Design review of the part built by this model. Coordinates are the model's own, in mm. A direction names the side the tool comes from. Give positions to 0.01 mm unless a question says otherwise; leave off trailing zeros. Loops run counter-clockwise (first coordinate to the right, second up) from the corner with the lowest first, then second, coordinate; pieces in that order, holes last.
Autodesk Inventor part; units mm, degrees
ref_plane "YZ Plane" through (0, 0, 0) normal (1, 0, 0) x (0, 1, 0)
ref_plane "XZ Plane" through (0, 0, 0) normal (0, 1, 0) x (-1, 0, 0)
ref_plane "XY Plane" through (0, 0, 0) normal (0, 0, 1) x (1, 0, 0)
sketch "Sketch1" plane through (0, 0, 0) normal (0, 1, 0) x (-1, 0, 0)
  line L0 (0, 0) -> (2500, 0)
  line L1 (2500, 0) -> (2500, -1250)
  line L2 (2500, -1250) -> (0, -1250)
  line L3 (0, -1250) -> (0, 0)
  dimension "d0" = 2500
  dimension "d1" = 1250
extrude "Extrusion1" add sketch "Sketch1" along normal blind 600
sketch "Sketch2" plane through (0, 0, 0) normal (0, -1, 0) x (1, 0, 0)
  line L0 (-50, -50) -> (-2450, -50)
  line L1 (-2450, -50) -> (-2450, -1200)
  line L2 (-2450, -1200) -> (-50, -1200)
  line L3 (-50, -1200) -> (-50, -50)
  line L4 (0, 0) -> (-2500, 0)
  line L5 (0, -1250) -> (0, 0)
  dimension "d4" = 2400
  dimension "d5" = 1150
  dimension "d8" = 50
  dimension "d9" = 50
  dimension "d10" = 2500
  dimension "d11" = 1250
extrude "Extrusion2" cut sketch "Sketch2" against normal blind 500
sketch "Sketch3" plane through (-2500, 0, 0) normal (0, 0, 1) x (1, 0, 0)
  line L0 (2500, 0) -> (0, 0)
  line L1 (2500, 0) -> (2500, 600)
  line L2 (0, 0) -> (0, 600)
  circle A0 centre (2476, 24) radius 4
  circle A1 centre (2460, 24) radius 4
  dimension "d12" = 8
  dimension "d13" = 24
  dimension "d14" = 24
  dimension "d20" = 8
  dimension "d21" = 24
  dimension "d23" = 16
extrude "Extrusion3" cut sketch "Sketch3" against normal blind 10
ref_plane "Work Plane1" through (-2500, 0, -625) normal (0, 0, 1) x (1, 0, 0)
mirror "Mirror1" about plane through (-2500, 0, -625) normal (0, 0, 1) of "Extrusion3"
ref_plane "Work Plane2" through (-1250, 0, -1250) normal (-1, 0, 0) x (0, 0, 1)
mirror "Mirror2" about plane through (-1250, 0, -1250) normal (-1, 0, 0) of "Extrusion3"
mirror "Mirror3" about plane through (-2500, 0, -625) normal (0, 0, 1) of "Mirror2", "Extrusion3"
equation "\"d0\" = 2 * d1"
equation "\"d4\" = d10 - 2 * d9"
equation "\"d5\" = d11 - 2 * d8"
equation "\"d9\" = d8"
equation "\"d13\" = 3 * d12"
equation "\"d14\" = 3 * d12"
equation "\"d20\" = d12"
equation "\"d21\" = d13"
equation "\"d23\" = 2 * d12"
properties part number "Base" material "Wood (Birch)"
Q1. Take a section at B-B (z = -1128.5). Give the boundary of the cut face in (x, y).
Results:
outline: (-2500, 0) - (-2450, 0) - (-2450, 500) - (-50, 500) - (-50, 0) - (0, 0) - (0, 600) - (-2500, 600) - close
Q2. Draft analysis for pull direction Z (two halves, no side actions). For faces 3 (the face through (-50, 246, -633)), 4 (the face through (-1267, 296, -1250)), 5 (the face through (-874, 0, -20)), 6 (the face through (-1233, 296, 0)), state which applies: pulls with the +Z half, pulls with the -Z half, needs draft (parallel to the pull), parting line crosses it, or undercut.
Results:
face 3: undercut
face 4: pulls with the -Z half
face 5: needs draft
face 6: pulls with the +Z half
Q3. Take a section at A-A (y = 393.5). Give the boundary of the cut face in (x, z).
Results:
outline: (-2500, -1250) - (0, -1250) - (0, 0) - (-2500, 0) - close; hole (-2450, -1200) - (-50, -1200) - (-50, -50) - (-2450, -50) - close
Q4. Take a section at C-C (x = -1752). Give the boundary of the cut face in (y, z).
Results:
outline: (0, -1250) - (600, -1250) - (600, 0) - (0, 0) - (0, -50) - (500, -50) - (500, -1200) - (0, -1200) - close
Q5. Tool access review of faces 1 (the face through (-1267, 246, -1200)), 2 (the face through (0, 296, -634)): name each direction out of +Z, -Z, +X, -X, +Y, -Y from which nothing blocks a thin tool from reaching the whole face with its end or side.
Results:
face 1: -Y
face 2: +Z, -Z, +X, +Y, -Y
Q6. Wall thickness on line 1 (Z direction, x = -432.5, y = 79.5); line 2 (Y direction, x = -2476, z = -1244); line 3 (X direction, y = 163, z = -478): over which ranges is each line inside the solid? List them lowest first.
Results:
line 1: z = -1250 to -1200, -50 to 0
line 2: y = 0 to 20, 28 to 600
line 3: x = -2500 to -2450, -50 to 0
Q7. Insertion check: pin 1 (2.5 mm diameter, centred on x = -23, y = 24, fed in from -Z); pin 2 (3 mm diameter, centred on x = -2076, z = -912, fed in from -Y); pin 3 (2.5 mm diameter, centred on x = -23, y = 23.5, fed in from +Z). Each pin has a flat end and moves straight along its axis. Give the tip position at first contact, or say it passes through.
Results:
pin 1: stops at z = -1240
pin 2: stops at y = 500
pin 3: stops at z = -10
